Here's how the part is built. I have some questions about the finished solid (model axes, mm). Coordinates: 2 decimals unless noted, no trailing zeros. Write each loop counter-clockwise with the first axis right and the second up, starting at its lowest first coordinate (ties: lowest second). Pieces come first, ordered by that corner, then holes.
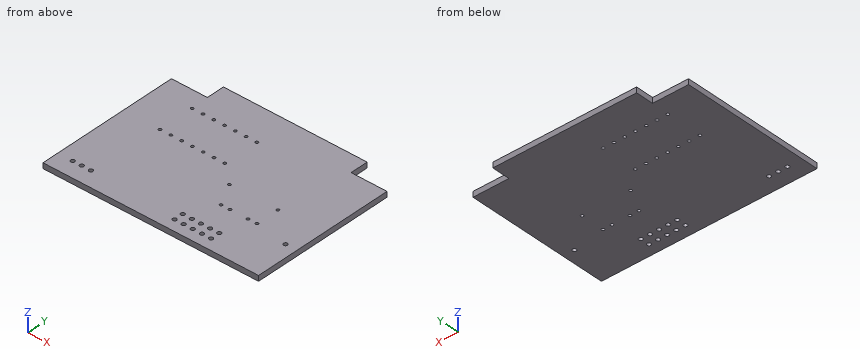
from build123d import *

# Parameters (mm, degrees)
EXTRUDE_1_DEPTH     = 1.5
SKETCH_2_R          = 0.55
CUT_EXTRUDE_1_DEPTH = 1.5
SKETCH_3_R          = 0.4
CUT_EXTRUDE_2_DEPTH = 10
SKETCH_6_R          = 0.4
CUT_EXTRUDE_4_DEPTH = 10
SKETCH_7_W          = 32.724153791
SKETCH_7_H          = 59.56032811
CUT_EXTRUDE_5_DEPTH = 10
SKETCH_8_R          = 0.55
CUT_EXTRUDE_6_DEPTH = 10


with BuildPart() as part:
    # Эскиз1 → Вытянуть1 (new body)
    with BuildSketch(Plane.XY):
        Polygon((0, 20), (0, 25), (40, 25), (40, 20), (50, 20), (50, -20), (-40, -20), (-40, 20), align=None)
    extrude(amount=EXTRUDE_1_DEPTH)

    # Эскиз2 → Вырез-Вытянуть1 (cut)
    with BuildSketch(Plane.XY.offset(1.5)):
        with Locations((-5.85, -15.4)):
            Circle(SKETCH_2_R)
        with Locations((-0.77, -15.4)):
            Circle(SKETCH_2_R)
        with Locations((-3.31, -15.4)):
            Circle(SKETCH_2_R)
        with Locations((23.75, -14.25)):
            Circle(SKETCH_2_R)
        with Locations((23.75, -16.79)):
            Circle(SKETCH_2_R)
        with Locations((26.29, -14.25)):
            Circle(SKETCH_2_R)
        with Locations((26.29, -16.79)):
            Circle(SKETCH_2_R)
        with Locations((28.83, -14.25)):
            Circle(SKETCH_2_R)
        with Locations((28.83, -16.79)):
            Circle(SKETCH_2_R)
        with Locations((31.37, -14.25)):
            Circle(SKETCH_2_R)
        with Locations((31.37, -16.79)):
            Circle(SKETCH_2_R)
        with Locations((33.91, -14.25)):
            Circle(SKETCH_2_R)
        with Locations((33.91, -16.79)):
            Circle(SKETCH_2_R)
    extrude(amount=-CUT_EXTRUDE_1_DEPTH, mode=Mode.SUBTRACT)

    # Эскиз3 → Вырез-Вытянуть2 (cut)
    with BuildSketch(Plane.XY.offset(1.5)):
        with Locations((37.5, -6.5)):
            Circle(SKETCH_3_R)
        with Locations((30, -6.5)):
            Circle(SKETCH_3_R)
        with Locations((0.25, 15)):
            Circle(SKETCH_3_R)
        with Locations((0.25, 5)):
            Circle(SKETCH_3_R)
        with Locations((3.25, 15)):
            Circle(SKETCH_3_R)
        with Locations((3.25, 5)):
            Circle(SKETCH_3_R)
        with Locations((6.25, 15)):
            Circle(SKETCH_3_R)
        with Locations((6.25, 5)):
            Circle(SKETCH_3_R)
        with Locations((9.25, 15)):
            Circle(SKETCH_3_R)
        with Locations((9.25, 5)):
            Circle(SKETCH_3_R)
        with Locations((12.25, 15)):
            Circle(SKETCH_3_R)
        with Locations((12.25, 5)):
            Circle(SKETCH_3_R)
        with Locations((15.25, 15)):
            Circle(SKETCH_3_R)
        with Locations((15.25, 5)):
            Circle(SKETCH_3_R)
        with Locations((18.25, 15)):
            Circle(SKETCH_3_R)
        with Locations((18.25, 5)):
            Circle(SKETCH_3_R)
        with Locations((35, -6.5)):
            Circle(SKETCH_3_R)
        with Locations((27.5, -6.5)):
            Circle(SKETCH_3_R)
    extrude(amount=-CUT_EXTRUDE_2_DEPTH, mode=Mode.SUBTRACT)

    # Эскиз6 → Вырез-Вытянуть4 (cut)
    with BuildSketch(Plane.XY.offset(1.5)):
        with Locations((24, 0)):
            Circle(SKETCH_6_R)
        with Locations((37.5, 0)):
            Circle(SKETCH_6_R)
    extrude(amount=-CUT_EXTRUDE_4_DEPTH, mode=Mode.SUBTRACT)

    # Эскиз7 → Вырез-Вытянуть5 (cut)
    with BuildSketch(Plane(origin=(0, 0, 0), x_dir=(-1, 0, 0), z_dir=(0, 0, -1))):
        with Locations((26.362076896, -0.829414575)):
            Rectangle(SKETCH_7_W, SKETCH_7_H)
    extrude(amount=-CUT_EXTRUDE_5_DEPTH, mode=Mode.SUBTRACT)

    # Эскиз8 → Вырез-Вытянуть6 (cut)
    with BuildSketch(Plane.XY.offset(1.5)):
        with Locations((46.8, -8)):
            Circle(SKETCH_8_R)
    extrude(amount=-CUT_EXTRUDE_6_DEPTH, mode=Mode.SUBTRACT)


solid = part.part
1. I want a section at A-A (z = 0.8). State how many separate pieces and enclosed holes the cut face has, then the cut area to 3 significant figures.
2. For pin 1 Ø0.8 at (y, z) = (23, 0.5) entering from +X, with a flat end and sliding along its axis, tell me the tip position at first contact or that it passes through.
3. If I drill on line 1 (Y direction, x = 18.25, z = 0.4); line 2 (Y direction, x = 31, z = 1.25); line 3 (X direction, y = -14, z = 0.45), over which ranges is the centre line in solid material (lowest first)?
4. I want a section at B-B (x = 43). List the corners of the cut face in (y, z) for me.
Response values:
1. separate pieces: 1
1. enclosed holes: 34
1. area: 2,580 mm2
2. pin 1: stops at x = 40
3. line 1: y = -20 to 4.6, 5.4 to 14.6, 15.4 to 25
3. line 2: y = -20 to -17.2, -16.38 to -14.66, -13.84 to 25
3. line 3: x = -10 to 23.26, 24.24 to 25.8, 26.78 to 28.34, 29.32 to 30.88, 31.86 to 33.42, 34.4 to 50
4. outline: (-20, 0) - (20, 0) - (20, 1.5) - (-20, 1.5) - close
